from build123d import *

# Parameters (mm, degrees)
BOSS_EXTRUDE1_DEPTH = 95.2
FILLET1_R           = 1
FILLET2_R           = 1
FILLET3_R           = 1
FILLET4_R           = 1
FILLET20_R          = 1
FILLET21_R          = 1
FILLET22_R          = 1
FILLET23_R          = 1


with BuildPart() as part:
    # Sketch1 → Boss-Extrude1 (new body)
    with BuildSketch(Plane(origin=(0, 0, 0), x_dir=(1, 0, 0), z_dir=(0, 1, 0))):
        with BuildLine():
            Line((-0.8, -0.8), (-0.8, -2.102974084))
            ThreePointArc((-0.8, -2.102974084), (0, -2.25), (0.8, -2.102974084))
            Line((0.8, -2.102974084), (0.8, -0.8))
            Line((0.8, -0.8), (2.102974084, -0.8))
            ThreePointArc((2.102974084, -0.8), (2.25, 0), (2.102974084, 0.8))
            Line((2.102974084, 0.8), (0.8, 0.8))
            Line((0.8, 0.8), (0.8, 2.102974084))
            ThreePointArc((0.8, 2.102974084), (0, 2.25), (-0.8, 2.102974084))
            Line((-0.8, 2.102974084), (-0.8, 0.8))
            Line((-0.8, 0.8), (-2.102974084, 0.8))
            ThreePointArc((-2.102974084, 0.8), (-2.25, 0), (-2.102974084, -0.8))
            Line((-2.102974084, -0.8), (-0.8, -0.8))
        make_face()
    extrude(amount=BOSS_EXTRUDE1_DEPTH)

    # Fillet1
    fillet1_edges = [part.edges().sort_by_distance(p)[0] for p in [
        (-2.25, 0, 0),
    ]]
    fillet(fillet1_edges, radius=FILLET1_R)

    # Fillet2
    fillet2_edges = [part.edges().sort_by_distance(p)[0] for p in [
        (0, 0, 2.25),
    ]]
    fillet(fillet2_edges, radius=FILLET2_R)

    # Fillet3
    fillet3_edges = [part.edges().sort_by_distance(p)[0] for p in [
        (2.25, 0, 0),
    ]]
    fillet(fillet3_edges, radius=FILLET3_R)

    # Fillet4
    fillet4_edges = [part.edges().sort_by_distance(p)[0] for p in [
        (0, 0, -2.25),
    ]]
    fillet(fillet4_edges, radius=FILLET4_R)

    # Fillet20
    fillet20_edges = [part.edges().sort_by_distance(p)[0] for p in [
        (2.25, 95.2, 0),
    ]]
    fillet(fillet20_edges, radius=FILLET20_R)

    # Fillet21
    fillet21_edges = [part.edges().sort_by_distance(p)[0] for p in [
        (0, 95.2, 2.25),
    ]]
    fillet(fillet21_edges, radius=FILLET21_R)

    # Fillet22
    fillet22_edges = [part.edges().sort_by_distance(p)[0] for p in [
        (-2.25, 95.2, 0),
    ]]
    fillet(fillet22_edges, radius=FILLET22_R)

    # Fillet23
    fillet23_edges = [part.edges().sort_by_distance(p)[0] for p in [
        (0, 95.2, -2.25),
    ]]
    fillet(fillet23_edges, radius=FILLET23_R)


solid = part.part
Could you check a few things on this model? Use its own coordinates, in mm. Coordinates: 2 decimals unless noted, no trailing zeros. Order: outer loops, then holes, each group sorted by start corner. A loop starts at its lowest first (then second) coordinate and runs counter-clockwise, first axis right, second up.
Q1. Suppose I cut it at A-A on y = 66. Please give me the cut outline in (x, z), and give its area (3 significant figures).
Q2. Please list where these lines run through material, in increasing order: L1, parallel to X at y = 12, z = 1; L2, parallel to Z at x = -0.1, y = 64.5.
Q3. Will these pins go through, and if not, where does the flat tip stop? pin 1 (0.7 mm diameter, centred on x = 1.5, y = 32.5, fed in from -Z); pin 2 (2 mm diameter, centred on x = 0.5, y = 28, fed in from -Z); pin 3 (1 mm diameter, centred on y = 57.5, z = 1.5, fed in from -X); pin 4 (1 mm diameter, centred on x = -1.5, y = 57.5, fed in from +Z).
Answer:
1. outline: (-2.1, -0.8) - (-0.8, -0.8) - (-0.8, -2.1) arc R2.25 ccw to (0.8, -2.1) - (0.8, -0.8) - (2.1, -0.8) arc R2.25 ccw to (2.1, 0.8) - (0.8, 0.8) - (0.8, 2.1) arc R2.25 ccw to (-0.8, 2.1) - (-0.8, 0.8) - (-2.1, 0.8) arc R2.25 ccw to start
1. area: 11.5 mm2
2. L1: x = -0.8 to 0.8
2. L2: z = -2.25 to 2.25
3. pin 1: stops at z = -0.8
3. pin 2: stops at z = -2.25
3. pin 3: stops at x = -0.8
3. pin 4: stops at z = 0.8
